Verification items for the finished model (mm, model axes). A direction names the side the tool comes from. Give positions to 0.01 mm unless a question says otherwise; leave off trailing zeros. Loops run counter-clockwise (first coordinate to the right, second up) from the corner with the lowest first, then second, coordinate; pieces in that order, holes last. Notation, with made-up numbers: M 34,87 L 71,87 A21 ccw 71,118 Z; hole C 52,63 d7. An arc over 180 degrees is marked long. Write each question's results on one line, items separated by ' | '. Start each with the question number.
Autodesk Inventor part; units mm, degrees
ref_plane "YZ Plane" through (0, 0, 0) normal (1, 0, 0) x (0, 1, 0)
ref_plane "XZ Plane" through (0, 0, 0) normal (0, 1, 0) x (-1, 0, 0)
ref_plane "XY Plane" through (0, 0, 0) normal (0, 0, 1) x (1, 0, 0)
sketch "スケッチ1" plane through (0, 0, 0) normal (0, 1, 0) x (-1, 0, 0)
  line L0 (11.25, 0) -> (-11.25, 0)
  line L1 (-11.25, 0) -> (-11.25, -120)
  line L2 (-11.25, -120) -> (11.25, -120)
  line L3 (11.25, -120) -> (11.25, 0)
  point P0 (0, 0)
  point P1 (0, 0)
  dimension "d0" = 22.5
  dimension "d3" = 120
extrude "押し出し1" add sketch "スケッチ1" along normal blind 2
sketch "スケッチ2" plane through (0, 0, 0) normal (0, -1, 0) x (1, 0, 0)
  line L0 (19, -120) -> (-19, -120)
  line L1 (-19, -120) -> (-19, -103.05)
  line L2 (-19, -103.05) -> (19, -103.05)
  line L3 (19, -103.05) -> (19, -120)
  line L4 (11.25, -120) -> (-11.25, -120)
  point P0 (0, 0)
  point P1 (0, -120)
  dimension "d6" = 38
  dimension "d11" = 16.95
extrude "押し出し2" add sketch "スケッチ2" against normal blind 13.44
sketch "スケッチ4" plane through (11.25, 0, -103.05) normal (0, 0, 1) x (1, 0, 0)
  circle A0 centre (-11.25, 20) radius 20
  line L0 (7.75, 0) -> (0, 0)
  line L1 (-22.5, 0) -> (0, 0)
  point P0 (-11.25, 0)
  point P1 (-11.25, 0)
  dimension "d12" = 40
extrude "押し出し4" cut sketch "スケッチ4" along normal through all
sketch "スケッチ5" plane through (11.25, 0, -103.05) normal (0, 0, 1) x (1, 0, 0)
  circle A0 centre (-11.25, 20) radius 20
  arc A1 (-11.25, 0) -> (-2.5322, 2) centre (-11.25, 20) ccw
  line L0 (-30.25, 13.44) -> (7.75, 13.44)
  line L1 (7.75, 13.44) -> (7.75, -5)
  line L2 (7.75, -5) -> (-30.25, -5)
  line L3 (-30.25, -5) -> (-30.25, 13.44)
  line L4 (7.75, 0) -> (7.75, 13.44)
  line L5 (7.75, 0) -> (0, 0)
  line L6 (-30.25, 4.22) -> (-11.25, 20)
  line L7 (-11.25, 20) -> (7.75, 4.22)
  point P0 (3.875, 0)
  point P1 (7.6436, 13.44)
  point P2 (-30.1436, 13.44)
  point P3 (7.75, 4.22)
  point P4 (4.1356, 7.2218)
  point P5 (-26.6356, 7.2218)
  point P6 (-3.3514, 13.44)
  point P7 (-19.1486, 13.44)
  dimension "d15" = 5
extrude "押し出し5" add sketch "スケッチ5" along normal up to surface (103.05 mm away) contours A0 L7 L1 L2 L3 L6
sketch "スケッチ24" plane through (11.25, 0, -103.05) normal (0, 0, -1) x (-1, 0, 0)
  line L0 (-7.75, 0) -> (11.25, 0)
  line L1 (-7.75, -5) -> (-7.75, 0)
  line L2 (30.25, -5) -> (-7.75, -5)
  line L3 (30.25, 0) -> (30.25, -5)
  line L4 (11.25, 0) -> (30.25, 0)
  point P0 (11.25, 0)
extrude "押し出し22" add sketch "スケッチ24" along normal up to surface (16.95 mm away)
sketch "スケッチ25" plane through (19, 13.44, -103.05) normal (1, 0, 0) x (0, 0, -1)
  line L0 (-103.05, -13.44) -> (-103.05, -6.2182)
  line L1 (16.95, -18.44) -> (16.95, 0)
  line L2 (16.95, -13.44) -> (-40.05, -13.44)
  line L3 (-40.05, -13.44) -> (-40.05, 1.46)
  line L4 (-40.05, 1.46) -> (16.95, 1.46)
  line L5 (16.95, 1.46) -> (16.95, -13.44)
  dimension "d77" = 14.9
  dimension "d78" = 57
extrude "押し出し23" add sketch "スケッチ25" against normal up to surface (38 mm away)
sketch "スケッチ26" plane through (19, -5, 0) normal (1, 0, 0) x (0, 0, -1)
  line L0 (63, 12.2218) -> (0, 12.2218)
  circle A0 centre (63, 12.2218) radius 12.2218
  line L1 (0, 0) -> (120, 0)
  circle A1 centre (84.1688, 0) radius 12.2218
  line L2 (84.1688, 12.2218) -> (120, 12.2218)
  line L3 (120, 0) -> (120, 19.9)
  point P0 (0, 5)
  point P1 (73.5844, 6.1109)
  point P2 (63, 0)
extrude "押し出し24" cut sketch "スケッチ26" against normal through all contours A1 L1 A0 | A1 L1 | L2 L3 L1 A1 picked at (80.2991, 4.512)
properties part number "arm_1_remake"
1. Set-up check for faces 1 (the face through (17.17, 5.74, -31.94)), 2 (the face through (0, 0, -32)), 3 (the face through (0, 7.222, -102)), 4 (the face through (-17.22, 5.7, -31.94)), 5 (the face through (0, 11, -120)): record each of +Z, -Z, +X, -X, +Y, -Y from which the full face is reachable in a straight line by a thin tool's end or side.
2. Section check C-C, the plane y = 5.25. Record the boundary of the cut face in (x, z), plus the area to 3 significant figures.
3. Depth check by flat-ended pin: pin 1 Ø8 at (x, y) = (4, 6) entering from +Z; pin 2 Ø2 at (y, z) = (4.5, -102.5) entering from +X; pin 3 Ø5 at (x, y) = (9, 2.5) entering from -Z; pin 4 Ø3 at (x, z) = (-4.5, -23) entering from +Y. Enter the tip coordinate at first touch or a pass-through.
4. Thickness scan on probe 1 along Z at (x, y) = (-7.5, 12); probe 2 along X at (y, z) = (6.25, -33); probe 3 along Y at (x, z) = (-8.5, -92.5). Record the ranges inside material, lowest first.
5. Section check D-D, the plane x = -9. Record the boundary of the cut face in (y, z), plus the area to 3 significant figures.
6. Section check A-A, the plane z = -27. Record the boundary of the cut face in (x, y), plus the area to 3 significant figures.
7. Section check B-B, the plane x = 4.5. Record the boundary of the cut face in (y, z), plus the area to 3 significant figures.
Filled sheet:
1) face 1: +Z, +X, +Y | face 2: +Z, +Y | face 3: -Z, +X, -X, -Y | face 4: +Z, -X, +Y | face 5: -Z, +X, -X, +Y, -Y
2) outline: M -19,-77.51 L 19,-77.51 L 19,-63 L 17.76,-63 L 17.76,0 L 13.51,0 L 13.51,-63 L -13.51,-63 L -13.51,0 L -17.76,0 L -17.76,-63 L -19,-63 Z | area: 1,090 mm2
3) pin 1: z = -63 | pin 2: through | pin 3: z = -77.14 | pin 4: y = 0.92
4) probe 1: -120 to -63 | probe 2: -16.56 to -14.52, 14.52 to 16.56 | probe 3: 7.22 to 14.9
5) outline: M -5,-63 A12.22 ccw 1.11,-73.58 A12.22 cw 7.22,-84.17 L 7.22,-120 L 14.9,-120 L 14.9,-63 L 2.14,-63 L 2.14,0 L -5,0 Z | area: 1,020 mm2
6) outline: M -19,-5 L 19,-5 L 19,4.22 L 15.39,7.22 A20 cw -15.39,7.22 L -19,4.22 Z | area: 299 mm2
7) outline: M -5,-63 A12.22 ccw 1.11,-73.58 A12.22 cw 7.22,-84.17 L 7.22,-120 L 14.9,-120 L 14.9,-63 L 0.51,-63 L 0.51,0 L -5,0 Z | area: 914 mm2
